Part model, mm, in its own coordinate system. A direction names the side the tool comes from. Give positions to 0.01 mm unless a question says otherwise; leave off trailing zeros. Order: outer loops, then holes, each group sorted by start corner. A loop starts at its lowest first (then second) coordinate and runs counter-clockwise, first axis right, second up. Notation, with made-up numbers: M 44,70.5 L 80,70.5 A25 cw 80,85.5 Z; hole C 87,87.5 d4. An arc over 180 degrees is marked long. Return JSON: item names as keys, results as strings.
from build123d import *

# Parameters (mm, degrees)
F1_DEPTH = 90


with BuildPart() as f1:
    # F0 (on Front) → F1 (new body)
    with BuildSketch(Plane.XZ):
        with BuildLine():
            Line((-15.323647, 22.809437), (-14.54678, 20.433205))
            ThreePointArc((-14.54678, 20.433205), (-31.205136, 6.918424), (-34.580102, -14.265527))
            Line((-34.580102, -14.265527), (-37.026413, -14.780856))
            ThreePointArc((-37.026413, -14.780856), (-33.3702, -24.331576), (-26.92714, -32.273309))
            Line((-26.92714, -32.273309), (-25.257697, -30.412407))
            ThreePointArc((-25.257697, -30.412407), (-5.224374, -38.081576), (14.808948, -30.412407))
            Line((14.808948, -30.412407), (16.478392, -32.273309))
            ThreePointArc((16.478392, -32.273309), (22.921451, -24.331576), (26.577664, -14.780856))
            Line((26.577664, -14.780856), (24.131354, -14.265527))
            ThreePointArc((24.131354, -14.265527), (23.091117, 1.829678), (13.866516, 15.060116))
            Line((13.866516, 15.060116), (13.326836, 14.405924))
            ThreePointArc((13.326836, 14.405924), (12.941248, 14.718539), (12.550393, 15.024543))
            Line((12.550393, 15.024543), (13.067485, 15.696731))
            ThreePointArc((13.067485, 15.696731), (12.659955, 16.004743), (12.247241, 16.30577))
            Line((12.247241, 16.30577), (11.753336, 15.616366))
            ThreePointArc((11.753336, 15.616366), (11.347366, 15.902013), (10.93659, 16.180706))
            Line((10.93659, 16.180706), (11.406734, 16.886528))
            ThreePointArc((11.406734, 16.886528), (10.979187, 17.166089), (10.546941, 17.43833))
            Line((10.546941, 17.43833), (10.101103, 16.716909))
            ThreePointArc((10.101103, 16.716909), (9.676632, 16.974263), (9.247842, 17.224353))
            Line((9.247842, 17.224353), (9.668858, 17.960536))
            ThreePointArc((9.668858, 17.960536), (9.223275, 18.210351), (8.773503, 18.452542))
            Line((8.773503, 18.452542), (8.377798, 17.70245))
            ThreePointArc((8.377798, 17.70245), (7.936796, 17.930319), (7.491979, 18.150645))
            Line((7.491979, 18.150645), (7.861915, 18.913776))
            ThreePointArc((7.861915, 18.913776), (7.400363, 19.132685), (6.93515, 19.343703))
            Line((6.93515, 19.343703), (6.591413, 18.568419))
            ThreePointArc((6.591413, 18.568419), (6.135926, 18.765745), (5.677145, 18.955287))
            Line((5.677145, 18.955287), (5.994285, 19.741826))
            ThreePointArc((5.994285, 19.741826), (5.051974, 20.103467), (4.098031, 20.433205))
            Line((4.098031, 20.433205), (4.874898, 22.809437))
            ThreePointArc((4.874898, 22.809437), (-0.111055, 24.013656), (-5.224374, 24.418424))
            ThreePointArc((-5.224374, 24.418424), (-10.337694, 24.013656), (-15.323647, 22.809437))
        make_face()
        with BuildLine():
            ThreePointArc((-12.993045, 15.680742), (-9.157697, 16.607064), (-5.224374, 16.918424))
            ThreePointArc((-5.224374, 16.918424), (-1.291052, 16.607064), (2.544297, 15.680742))
            Line((2.544297, 15.680742), (3.165791, 17.581727))
            ThreePointArc((3.165791, 17.581727), (18.158312, 5.418424), (21.195781, -13.647132))
            Line((21.195781, -13.647132), (19.238732, -13.234869))
            ThreePointArc((19.238732, -13.234869), (16.426261, -20.581576), (11.470061, -26.690602))
            Line((11.470061, -26.690602), (12.805616, -28.179324))
            ThreePointArc((12.805616, -28.179324), (-5.224374, -35.081576), (-23.254364, -28.179324))
            Line((-23.254364, -28.179324), (-21.91881, -26.690602))
            ThreePointArc((-21.91881, -26.690602), (-26.875009, -20.581576), (-29.687481, -13.234869))
            Line((-29.687481, -13.234869), (-31.644529, -13.647132))
            ThreePointArc((-31.644529, -13.647132), (-28.60706, 5.418424), (-13.614539, 17.581727))
            Line((-13.614539, 17.581727), (-12.993045, 15.680742))
        make_face(mode=Mode.SUBTRACT)
    extrude(amount=F1_DEPTH)


solid = f1.part
Q1. Two-plate mould, pull along X, no slides. Class faces 5 (the cylindrical face through (16.48, -44.37, -20.49)), 6 (the flat face through (13.5, -90, -25.2)), 7 (the cylindrical face through (-31.05, -44.37, 7.184)), 8 (the cylindrical face through (22.849, -44.37, -24.456)): +X half, -X half, draft (parallel to the pull), parting line (faces both ways), or undercut.
Established:
{"face 5": "undercut", "face 6": "draft", "face 7": "-X half", "face 8": "+X half"}
Q2. 3-axis set-ups, long thin cutter, end or side, ignore diameter. For faces 1 (the flat face through (20.231, -44.37, -13.444)), 2 (the cylindrical face through (-33.44, -44.37, -24.21)), 3 (the flat face through (-35.79, -44.37, -14.52)), 4 (the flat face through (4.48, -44.37, 21.6)): which of +Z, -Z, +X, -X, +Y, -Y reach the whole face in a straight line?
Established:
{"face 1": "+Y, -Y", "face 2": "-Z, -X, +Y, -Y", "face 3": "-X, +Y, -Y", "face 4": "+X, +Y, -Y"}
Q3. Band-saw the part on B-B (x = 18). Give the cut face in (y, z), then the cut area to 3 significant figures.
Established:
{"outline": "M -90,-30.82 L 0,-30.82 L 0,-17.34 L -90,-17.34 Z; M -90,5.69 L 0,5.69 L 0,10.91 L -90,10.91 Z", "area": "1,680 mm²"}
Q4. Pin check, flat tips, straight feed: pin 1 (8 mm diameter, centred on x = 12, z = 0.5, fed in from -Y); pin 2 (10 mm diameter, centred on y = -59, z = 2.5, fed in from +X); pin 3 (1 mm diameter, centred on x = 6, y = -53, fed in from -Z); pin 4 (6 mm diameter, centred on y = -35.5, z = 11.5, fed in from +X). Stop position of each tip, or through.
Established:
{"pin 1": "passes through", "pin 2": "stops at x = 24.25", "pin 3": "stops at z = -36.1", "pin 4": "stops at x = 19.78"}
Q5. Probe line 1 along Z through (x, y) = (-17, -30); line 2 along Z through (x, y) = (2, -27); line 3 along X through (y, z) = (-49.5, 5). List the from-to ranges inside material, lowest first.
Established:
{"line 1": "z = -35.67 to -32.38, 16.22 to 19.51", "line 2": "z = -37.2 to -34.1, 15.85 to 23.61", "line 3": "x = -32.22 to -28.84, 18.39 to 21.77"}
Q6. Band-saw the part on A-A (z = -0.5). Give the cut face in (x, y).
Established:
{"outline": "M -34.25,-90 L -31.14,-90 L -31.14,0 L -34.25,0 Z; M 20.69,-90 L 23.8,-90 L 23.8,0 L 20.69,0 Z"}
